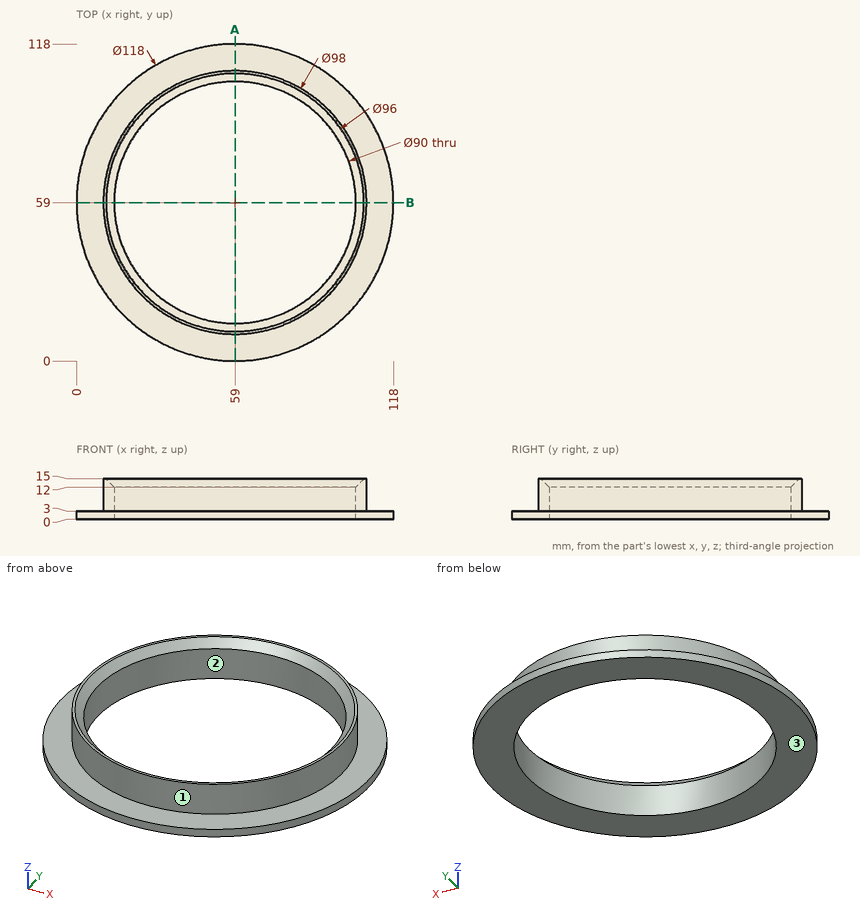
Verification items for this drawing (mm, ordinates from the low corner). Coordinates: 2 decimals unless noted, no trailing zeros. Order: outer loops, then holes, each group sorted by start corner. A loop starts at its lowest first (then second) coordinate and runs counter-clockwise, first axis right, second up. Notation, with made-up numbers: M 16.5,15.5 L 74.5,15.5 A16 ccw 74.5,23.5 Z; hole C 19.5,6 d9. An arc over 180 degrees is marked long. Use CSV: the item, a comma, the result in double quotes.
Item 1: Gauge pin test, flat ends, axial feed: pin 1 Ø8 at (x, z) = (48.5, 12.5) entering from +Y; pin 2 Ø8 at (y, z) = (16.5, 10.5) entering from +X; pin 3 Ø1 at (y, z) = (53.5, 1.5) entering from +X; pin 4 Ø12 at (x, y) = (103.5, 67.5) entering from +Z. Record the tip position at first contact, or that the pin passes through.
Returned:
pin 1,"stops at y = 107.57"
pin 2,"stops at x = 89.31"
pin 3,"stops at x = 117.79"
pin 4,"stops at z = 15"
Item 2: Thickness scan on line 1 along Y through (x, z) = (59, 8); line 2 along Y through (x, z) = (27, 14.5); line 3 along Z through (x, y) = (113, 57). Record the ranges inside material, lowest first.
Returned:
line 1,"y = 10 to 14, 104 to 108"
line 2,"y = 21.89 to 23.9, 94.1 to 96.11"
line 3,"z = 0 to 3"
Item 3: Mould release check, pull along Y, two halves, no side actions. Record for the marked faces 1, 2 and 3: pulls with the +Y half, pulls with the -Y half, needs draft (parallel to the pull), parting line crosses it, or undercut.
Returned:
face 1,"parting line crosses it"
face 2,"undercut"
face 3,"needs draft"
Item 4: Cross-section at A-A on x = 59. Record the cut outline in (y, z).
Returned:
outline,"M 0,0 L 14,0 L 14,12 L 11,15 L 10,15 L 10,3 L 0,3 Z; M 104,0 L 118,0 L 118,3 L 108,3 L 108,15 L 107,15 L 104,12 Z"
